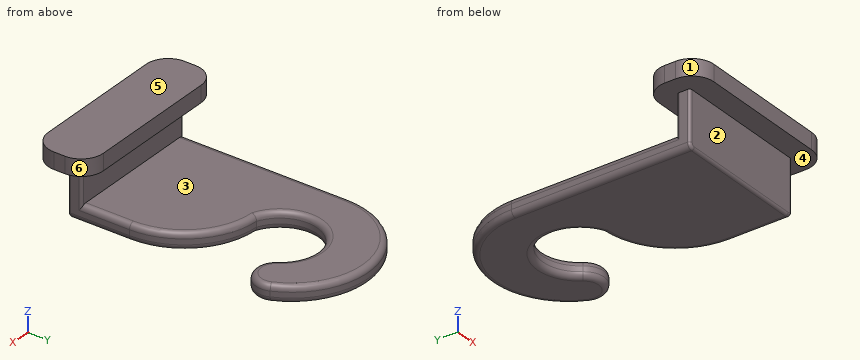
from build123d import *

# Parameters (mm, degrees)
F0_W     = 25
F0_H     = 3.598708484
F0_H_2   = 2.5
F1_DEPTH = 3
F2_DEPTH = 10
F3_START = 10
F3_DEPTH = 3
F4_R     = 4
F5_R     = 1
F6_R     = 0.5


with BuildPart() as f1:
    # F0 (on Top) → F1 (new body)
    with BuildSketch(Plane.XY):
        with BuildLine():
            Line((-12.0194856117, 31.2152840197), (-12.0194856117, 4.7718174662))
            Line((-12.0194856117, 4.7718174662), (12.9805143883, 4.7718174662))
            Line((12.9805143883, 4.7718174662), (12.9805143883, 9.8692406903))
            ThreePointArc((12.9805143883, 9.8692406903), (9.2091630199, 19.2346795626), (0, 23.3730189502))
            ThreePointArc((0, 23.3730189502), (-2.5235742208, 33.9593593839), (8.340984877, 33.3265985788))
            ThreePointArc((8.340984877, 33.3265985788), (13.0836829302, 32.1289610754), (14.685023576, 36.750998348))
            ThreePointArc((14.685023576, 36.750998348), (-0.9201685744, 44.8514028231), (-12.0194856117, 31.2152840197))
        make_face()
        with Locations((0.4805143883, 2.9724632242)):
            Rectangle(F0_W, F0_H)
        with Locations((0.4805143883, -0.0768910178)):
            Rectangle(F0_W, F0_H_2)
    extrude(amount=F1_DEPTH)

    # F0 (on Top) → F2 (join)
    with BuildSketch(Plane.XY):
        with Locations((0.4805143883, -0.0768910178)):
            Rectangle(F0_W, F0_H_2)
    extrude(amount=F2_DEPTH)

    # F0 (on Top) → F3 (join)
    with BuildSketch(Plane.XY.offset(F3_START)):
        with Locations((0.4805143883, 2.9724632242)):
            Rectangle(F0_W, F0_H)
        Polygon((-12.0194856117, -1.3268910178), (-12.0194856117, 1.1731089822), (-12.0194856117, 4.7718174662), (-15.4697376937, 4.7718174662), (-15.4697376937, -5.2281825338), (16.5302623063, -5.2281825338), (16.5302623063, 4.7718174662), (12.9805143883, 4.7718174662), (12.9805143883, 1.1731089822), (12.9805143883, -1.3268910178), align=None)
        with Locations((0.4805143883, -0.0768910178)):
            Rectangle(F0_W, F0_H_2)
    extrude(amount=F3_DEPTH)

    # F4
    f4_edges = [f1.edges().sort_by_distance(p)[0] for p in [
        (16.530262, -5.228183, 11.5),
        (16.530262, 4.771817, 11.5),
        (-15.469738, -5.228183, 11.5),
        (-15.469738, 4.771817, 11.5),
    ]]
    fillet(f4_edges, radius=F4_R)

    # F5
    f5_edges = [f1.edges().sort_by_distance(p)[0] for p in [
        (-2.523574, 33.959359, 3),
        (9.209163, 19.23468, 3),
        (12.980514, 5.521175, 3),
        (-0.920169, 44.851403, 0),
        (13.083683, 32.128961, 0),
        (-2.523574, 33.959359, 0),
        (9.209163, 19.23468, 0),
        (12.980514, 4.271175, 0),
        (-12.019486, 14.944197, 0),
    ]]
    fillet(f5_edges, radius=F5_R)

    # F6
    f6_edges = [f1.edges().sort_by_distance(p)[0] for p in [
        (12.980514, 1.173109, 6.5),
        (-12.019486, 1.173109, 6.5),
        (-12.019486, -1.326891, 5.5),
    ]]
    fillet(f6_edges, radius=F6_R)


solid = f1.part
Check sheet for the modelled part. Datum: model origin and axes. Units: mm. Face numbers are marked on the shaded views. A direction names the side the tool comes from. Give positions to 0.01 mm unless a question says otherwise; leave off trailing zeros. Loops run counter-clockwise (first coordinate to the right, second up) from the corner with the lowest first, then second, coordinate; pieces in that order, holes last. Notation, with made-up numbers: M 85.5,-31.75 L 109.5,-31.75 A26 cw 109.5,-6.75 Z; hole C 1,-18.75 d9. An arc over 180 degrees is marked long. Use a Markdown table: item, result. Add a question column.
Q1. Sectioned sample at B-B, the plane y = 7.5. Record the cut outline in (x, z), then the cut area to 3 significant figures.
Q2. Sectioned sample at A-A, the plane z = 5.25. Record the cut outline in (x, y).
Q3. Scan lines: line 1 along Z through (x, y) = (1, 3); line 2 along Z through (x, y) = (-6, 26); line 3 along Y through (x, z) = (-11, 6). Record each from-to range of solid material in increasing order. Write a range as [from, to].
Q4. Go/stop test with flat-tipped pins: pin 1 (3.5 mm diameter, centred on x = -3.5, z = 11.5, fed in from +Y); pin 2 (5 mm diameter, centred on x = -8.5, z = 6, fed in from +Y); pin 3 (5 mm diameter, centred on x = 1, z = 6.5, fed in from -Y). Record where each tip stops, or that it passes through.
Q5. Tool access check on the marked faces 1, 2 and 3. Record the directions out of +Z, -Z, +X, -X, +Y, -Y that give a thin tool (end or side, any length) a straight path to the whole face; none if there is none.
Q6. Mould release check, pull along Z, two halves, no side actions. Record for the marked faces 4, 5 and 6: pulls with the +Z half, pulls with the -Z half, needs draft (parallel to the pull), parting line crosses it, or undercut.
Verdict:
| question | item | result |
|---|---|---|
| 1 | outline | M -12.02,1 A1 ccw -11.02,0 L 11.98,0 A1 ccw 12.98,1 L 12.98,2 A1 ccw 11.98,3 L -11.02,3 A1 ccw -12.02,2 Z |
| 1 | area | 74.1 mm^2 |
| 2 | outline | M -12.02,-0.83 A0.5 ccw -11.52,-1.33 L 12.48,-1.33 A0.5 ccw 12.98,-0.83 L 12.98,0.67 A0.5 ccw 12.48,1.17 L -11.52,1.17 A0.5 ccw -12.02,0.67 Z |
| 3 | line 1 | [0, 3], [10, 13] |
| 3 | line 2 | [0, 3] |
| 3 | line 3 | [-1.33, 1.17] |
| 4 | pin 1 | y = 4.77 |
| 4 | pin 2 | y = 1.17 |
| 4 | pin 3 | y = -1.33 |
| 5 | face 1 | +Z, -Z, -X, -Y |
| 5 | face 2 | -Z, +X, -X, -Y |
| 5 | face 3 | +X, -X, +Y |
| 6 | face 4 | undercut |
| 6 | face 5 | pulls with the +Z half |
| 6 | face 6 | needs draft |
